```python
from build123d import *

# Parameters (mm, degrees)
BOSS_EXTRUDE1_DEPTH     = 5
CIRPATTERN1_COUNT       = 12
SKETCH4_R               = 16.811989879
SKETCH4_R_2             = 10.314619087
CUT_EXTRUDE1_DEPTH      = 0.5
SKETCH5_R               = 6.950731161
CUT_EXTRUDE2_DEPTH      = 46.5
CUT_EXTRUDE3_DEPTH      = 46.5
CIRPATTERN2_COUNT       = 12
CUT_EXTRUDE4_DEPTH      = 46.5
CUT_EXTRUDE4_DEPTH_BACK = 46.5
SKETCH10_W              = 3.744348286
SKETCH10_H              = 1.553508974


with BuildPart() as part:
    # Sketch1 → Boss-Extrude1 (new, symmetric)
    with BuildSketch(Plane.XY):
        with BuildLine():
            Line((2.932850173, 0), (-2.932850173, 0))
            Line((-2.932850173, 0), (-2.932850173, -21.812004013))
            ThreePointArc((-2.932850173, -21.812004013), (-1.626916196, -23.842475136), (-0.986171591, -26.170075379))
            ThreePointArc((-0.986171591, -26.170075379), (0, -26.142264995), (0.986171591, -26.170075379))
            ThreePointArc((0.986171591, -26.170075379), (1.626916196, -23.842475136), (2.932850173, -21.812004013))
            Line((2.932850173, -21.812004013), (2.932850173, 0))
        make_face()
        with BuildLine():
            ThreePointArc((-0.986171591, 26.170075379), (-1.626916196, 23.842475136), (-2.932850173, 21.812004013))
            Line((-2.932850173, 21.812004013), (-2.932850173, 0))
            Line((-2.932850173, 0), (2.932850173, 0))
            Line((2.932850173, 0), (2.932850173, 21.812004013))
            ThreePointArc((2.932850173, 21.812004013), (1.626916196, 23.842475136), (0.986171591, 26.170075379))
            ThreePointArc((0.986171591, 26.170075379), (0, 26.142264995), (-0.986171591, 26.170075379))
        make_face()
    boss_extrude1 = extrude(amount=BOSS_EXTRUDE1_DEPTH, both=True)

    # CirPattern1: Boss-Extrude1 ×12 about axis
    cirpattern1_axis = Axis((-1000, 0, 0), (1, 0, 0))
    for i in range(1, CIRPATTERN1_COUNT):
        add(boss_extrude1.rotate(cirpattern1_axis, i * 360 / CIRPATTERN1_COUNT))

    # Sketch4 → Cut-Extrude1 (cut)
    with BuildSketch(Plane.ZY.offset(2.932850173)):
        Circle(SKETCH4_R)
        Circle(SKETCH4_R_2, mode=Mode.SUBTRACT)
    cut_extrude1 = extrude(amount=-CUT_EXTRUDE1_DEPTH, mode=Mode.SUBTRACT)

    # Sketch5 → Cut-Extrude2 (cut)
    with BuildSketch(Plane.ZY.offset(2.932850173)):
        Circle(SKETCH5_R)
    cut_extrude2 = extrude(amount=-CUT_EXTRUDE2_DEPTH, mode=Mode.SUBTRACT)

    # Sketch6 → Cut-Extrude3 (cut)
    with BuildSketch(Plane.ZY.offset(2.932850173)):
        with BuildLine():
            Line((-26.170075379, -5), (-18.975291906, -3.625379681))
            ThreePointArc((-18.975291906, -3.625379681), (-18.830320626, -4.315565534), (-18.660254038, -5))
            Line((-18.660254038, -5), (-26.170075379, -5))
        make_face()
        with BuildLine():
            Line((-26.170075379, 5), (-18.975291906, 3.625379681))
            ThreePointArc((-18.975291906, 3.625379681), (-18.830320626, 4.315565534), (-18.660254038, 5))
            Line((-18.660254038, 5), (-26.170075379, 5))
        make_face()
    cut_extrude3 = extrude(amount=-CUT_EXTRUDE3_DEPTH, mode=Mode.SUBTRACT)

    # CirPattern2: Cut-Extrude3 ×12 about axis
    cirpattern2_axis = Axis((0, 0, 0), (1, 0, 0))
    for i in range(1, CIRPATTERN2_COUNT):
        add(cut_extrude3.rotate(cirpattern2_axis, i * 360 / CIRPATTERN2_COUNT), mode=Mode.SUBTRACT)

    # Sketch10 → Cut-Extrude4 (cut, two sides: drawn at the far end of the back side and taken through both)
    with BuildSketch(Plane.ZY.offset(2.432850173).offset(-CUT_EXTRUDE4_DEPTH_BACK)):
        with Locations((0, 6.950731161)):
            Rectangle(SKETCH10_W, SKETCH10_H)
    extrude(amount=CUT_EXTRUDE4_DEPTH + CUT_EXTRUDE4_DEPTH_BACK, mode=Mode.SUBTRACT)

    # Mirror3: Cut-Extrude1, Cut-Extrude2 across plane
    add(cut_extrude1.mirror(Plane(origin=(0, 0, 0), x_dir=(0, 0, 1), z_dir=(1, 0, 0))), mode=Mode.SUBTRACT)
    add(cut_extrude2.mirror(Plane(origin=(0, 0, 0), x_dir=(0, 0, 1), z_dir=(1, 0, 0))), mode=Mode.SUBTRACT)


solid = part.part
```
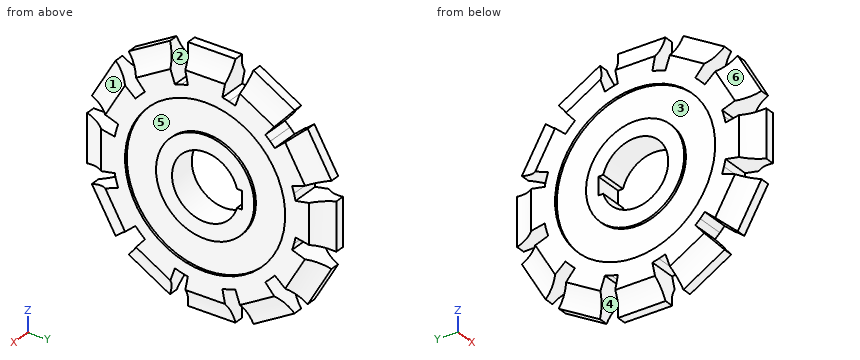
Can you work these out from the model? Positions are in its coordinate system, mm. Face numbers are marked on the shaded views. A direction names the side the tool comes from. Coordinates: 2 decimals unless noted, no trailing zeros. Loops run counter-clockwise (first coordinate to the right, second up) from the corner with the lowest first, then second, coordinate; pieces in that order, holes last.
1) For pin 1 (2 mm diameter, centred on x = 0.5, z = -10, fed in from -Y); pin 2 (4 mm diameter, centred on y = 10.5, z = -7, fed in from -X); pin 3 (3 mm diameter, centred on y = -14.5, z = 3, fed in from +X), each with a flat end and sliding along its axis, tell me the tip position at first contact or that it passes through.
2) Which directions (+Z, -Z, +X, -X, +Y, -Y) give clear straight access to the entire face, cutting with the end or side of a thin tool? Please do the marked faces 1, 2 and 3.
3) Imagine slicing it at B-B on z = 0. List the corners of the cut face in (x, y) for me, plus the area to 3 significant figures.
4) Imagine slicing it at A-A on y = 0. List the corners of the cut face in (x, z) for me.
5) I need wall thicknesses on probe 1 along Z at (x, y) = (0.25, 21.5); probe 2 along Y at (x, z) = (-0.25, -21); probe 3 along Y at (x, z) = (-2.65, 0). Which ranges of each line are inside material? Lowest first, please.
6) Thinking about a two-plate mould opening in Z: for the marked faces 4, 5 and 6, which applies, pulls with the +Z half, pulls with the -Z half, needs draft (parallel to the pull), parting line crosses it, or undercut?
Completed:
1. pin 1: stops at y = -25
1. pin 2: stops at x = -2.43
1. pin 3: stops at x = 2.43
2. face 1: +Z, +X, -Y
2. face 2: +Z, +X, -X
2. face 3: -X
3. outline: (-2.93, -21.81) arc R8 cw to (-0.99, -26.17) arc R17.5 cw to (0.99, -26.17) arc R8 cw to (2.93, -21.81) - (2.93, -16.81) - (2.43, -16.81) - (2.43, -10.31) - (2.93, -10.31) - (2.93, -6.95) - (-2.93, -6.95) - (-2.93, -10.31) - (-2.43, -10.31) - (-2.43, -16.81) - (-2.93, -16.81) - close; (-2.93, 7.73) - (2.93, 7.73) - (2.93, 10.31) - (2.43, 10.31) - (2.43, 16.81) - (2.93, 16.81) - (2.93, 21.81) arc R8 cw to (0.99, 26.17) arc R17.5 cw to (-0.99, 26.17) arc R8 cw to (-2.93, 21.81) - (-2.93, 16.81) - (-2.43, 16.81) - (-2.43, 10.31) - (-2.93, 10.31) - close
3. area: 186 mm2
4. outline: (-2.93, -21.81) arc R8 cw to (-0.99, -26.17) arc R17.5 cw to (0.99, -26.17) arc R8 cw to (2.93, -21.81) - (2.93, -16.81) - (2.43, -16.81) - (2.43, -10.31) - (2.93, -10.31) - (2.93, -6.95) - (-2.93, -6.95) - (-2.93, -10.31) - (-2.43, -10.31) - (-2.43, -16.81) - (-2.93, -16.81) - close; (-2.93, 6.95) - (2.93, 6.95) - (2.93, 10.31) - (2.43, 10.31) - (2.43, 16.81) - (2.93, 16.81) - (2.93, 21.81) arc R8 cw to (0.99, 26.17) arc R17.5 cw to (-0.99, 26.17) arc R8 cw to (-2.93, 21.81) - (-2.93, 16.81) - (-2.43, 16.81) - (-2.43, 10.31) - (-2.93, 10.31) - close
5. probe 1: z = -15.05 to -7.48, -4.11 to 4.11, 7.48 to 15.05
5. probe 2: y = -15.92 to -7.31, -4.01 to 4.01, 7.31 to 15.92
5. probe 3: y = -22.15 to -16.81, -10.31 to -6.95, 7.73 to 10.31, 16.81 to 22.15
6. face 4: pulls with the -Z half
6. face 5: undercut
6. face 6: pulls with the +Z half
